Verification items for the finished model (mm, model axes). A direction names the side the tool comes from. Coordinates: 2 decimals unless noted, no trailing zeros. Loops run counter-clockwise (first coordinate to the right, second up) from the corner with the lowest first, then second, coordinate; pieces in that order, holes last.
Q1. Go/stop test with flat-tipped pins: P1, Ø19.5, axis at x = -7.5, y = 12, coming from the -Z side; P2, Ø6, axis at x = 42, z = 45, coming from the +Y side; P3, Ø12, axis at x = 10, y = 7.5, coming from the +Z side. Record where each tip stops, or that it passes through.
Q2. Mould release check, pull along Y, two halves, no side actions. Record for faces 1 (the face through (52.598, -32, 32)), 2 (the face through (-48.03, -17.81, 48.24)), 3 (the face through (42, 30.4, 29)): +Y half, -Y half, draft (parallel to the pull), parting line (faces both ways), or undercut.
Q3. Sectioned sample at D-D (x = -43.5). Enter the section's corners in (y, z), then the cut area to 3 significant figures.
Q4. Material ranges on probe 1 along Y at (x, z) = (28, 30.4); probe 2 along Y at (x, z) = (12.5, 29.4); probe 3 along Y at (x, z) = (39, 27.5), recorded low to high.
Q5. Sectioned sample at C-C (z = 55). Enter the section's corners in (x, y).
Q6. Sectioned sample at B-B (y = -0.65). Enter the section's corners in (x, z), then the cut area to 3 significant figures.
Q7. Sectioned sample at A-A (x = -3). Enter the section's corners in (y, z).
Q8. Access from +Z, -Z, +X, -X, +Y, -Y to the whole of each face (thin tool, end or side, straight path). Record for faces 4 (the face through (-1, -32, 65)), 5 (the face through (-1, -6.3, 29)), 6 (the face through (25, 15, 29)).
```python
from build123d import *

# Parameters (mm, degrees)
EXTRUDE_7_DEPTH     = 65
SKETCH_6_W          = 4
SKETCH_6_H          = 4
EXTRUDE_10_DEPTH    = 65
SKETCH_7_W          = 4
SKETCH_7_H          = 42.3
EXTRUDE_11_DEPTH    = 92
SKETCH_8_R          = 11.5
CUT_EXTRUDE_2_DEPTH = 2
SKETCH_10_R         = 2.5
CUT_EXTRUDE_3_DEPTH = 2
SKETCH_11_R         = 1.5
CUT_EXTRUDE_6_DEPTH = 4
EXTRUDE_13_DEPTH    = 2
SKETCH_14_R         = 0.7
EXTRUDE_14_DEPTH    = 5


with BuildPart() as part:
    # 草图1 → 凸台-拉伸7 (new body)
    with BuildSketch(Plane.XY):
        Polygon((-50, -29), (-50, -30.5), (-52.598076211, -29), (-52.598076211, -34), (-50, -32.5), (-50, -35.5), (50, -35.5), (50, -32.5), (52.598076211, -34), (52.598076211, -29), (50, -30.5), (50, -29), align=None)
    extrude(amount=EXTRUDE_7_DEPTH)

    # 草图6 → 凸台-拉伸10 (add)
    with BuildSketch(Plane(origin=(0, -29, 0), x_dir=(1, 0, 0), z_dir=(0, 1, 0))):
        with Locations((-48, -29)):
            Rectangle(SKETCH_6_W, SKETCH_6_H)
    extrude_10 = extrude(amount=EXTRUDE_10_DEPTH)

    # 镜向1: 凸台-拉伸10 across plane
    add(extrude_10.mirror(Plane(origin=(0, 0, 0), x_dir=(0, 0, 1), z_dir=(1, 0, 0))))

    # 草图7 → 凸台-拉伸11 (add)
    with BuildSketch(Plane(origin=(-46, 0, 0), x_dir=(0, 0, -1), z_dir=(1, 0, 0))):
        with Locations((-29, 14.85)):
            Rectangle(SKETCH_7_W, SKETCH_7_H)
    extrude(amount=EXTRUDE_11_DEPTH)

    # 草图8 → 切除-拉伸2 (cut)
    with BuildSketch(Plane.XY.offset(31)):
        with Locations((-28, 14.85)):
            Circle(SKETCH_8_R)
        with Locations((28, 14.85)):
            Circle(SKETCH_8_R)
    extrude(amount=-CUT_EXTRUDE_2_DEPTH, mode=Mode.SUBTRACT)

    # 草图10 → 切除-拉伸3 (cut)
    with BuildSketch(Plane.XY.offset(29)):
        with Locations((-28, 14.85)):
            Circle(SKETCH_10_R)
        with Locations((28, 14.85)):
            Circle(SKETCH_10_R)
    extrude(amount=-CUT_EXTRUDE_3_DEPTH, mode=Mode.SUBTRACT)

    # 草图11 → 切除-拉伸6 (cut)
    with BuildSketch(Plane.XY.offset(31)):
        with Locations((-43.5, 30.35)):
            Circle(SKETCH_11_R)
        with Locations((-12.5, 30.35)):
            Circle(SKETCH_11_R)
        with Locations((-43.5, -0.65)):
            Circle(SKETCH_11_R)
        with Locations((-12.5, -0.65)):
            Circle(SKETCH_11_R)
        with Locations((12.5, 30.35)):
            Circle(SKETCH_11_R)
        with Locations((43.5, 30.35)):
            Circle(SKETCH_11_R)
        with Locations((12.5, -0.65)):
            Circle(SKETCH_11_R)
        with Locations((43.5, -0.65)):
            Circle(SKETCH_11_R)
    extrude(amount=-CUT_EXTRUDE_6_DEPTH, mode=Mode.SUBTRACT)

    # 草图13 → 凸台-拉伸13 (add, symmetric)
    with BuildSketch(Plane(origin=(48, 0, 0), x_dir=(0, 0, -1), z_dir=(1, 0, 0))):
        Polygon((-65, -29), (-31, -6.3), (-31, -11.3), (-57.511013216, -29), align=None)
    extrude_13 = extrude(amount=EXTRUDE_13_DEPTH, both=True)

    # 镜向3: 凸台-拉伸13 across plane
    add(extrude_13.mirror(Plane(origin=(0, 0, 0), x_dir=(0, 0, 1), z_dir=(1, 0, 0))))

    # 草图14 → 凸台-拉伸14 (add)
    with BuildSketch(Plane(origin=(0, -29, 0), x_dir=(1, 0, 0), z_dir=(0, 1, 0))):
        with Locations(Location((-30.407474137, -14.090366943, 0), (0, 0, 180))):
            Circle(SKETCH_14_R)
        with Locations(Location((-31.677474137, -62.350366943, 0), (0, 0, 180))):
            Circle(SKETCH_14_R)
        with Locations(Location((20.392525863, -29.330366943, 0), (0, 0, 180))):
            Circle(SKETCH_14_R)
        with Locations(Location((20.392525863, -57.270366943, 0), (0, 0, 180))):
            Circle(SKETCH_14_R)
    extrude(amount=EXTRUDE_14_DEPTH)


solid = part.part
```
Geometry check:
1. P1: stops at z = 27
1. P2: stops at y = -29
1. P3: stops at z = 31
2. face 1: draft
2. face 2: +Y half
2. face 3: undercut
3. outline: (-35.5, 0) - (-29, 0) - (-29, 65) - (-35.5, 65) - close; (-6.3, 27) - (-2.15, 27) - (-2.15, 31) - (-6.3, 31) - close; (0.85, 27) - (28.85, 27) - (28.85, 31) - (0.85, 31) - close; (31.85, 27) - (36, 27) - (36, 31) - (31.85, 31) - close
3. area: 568 mm2
4. probe 1: y = -35.5 to -29, -6.3 to 3.35, 26.35 to 36
4. probe 2: y = -35.5 to -29, -6.3 to -2.15, 0.85 to 28.85, 31.85 to 36
4. probe 3: y = -35.5 to -29, -6.3 to 36
5. outline: (-52.6, -34) - (-50, -32.5) - (-50, -35.5) - (50, -35.5) - (50, -32.5) - (52.6, -34) - (52.6, -29) - (50, -30.5) - (50, -29) - (-50, -29) - (-50, -30.5) - (-52.6, -29) - close; (-50, -27.32) - (-46, -27.32) - (-46, -22.32) - (-50, -22.32) - close; (46, -27.32) - (50, -27.32) - (50, -22.32) - (46, -22.32) - close
6. outline: (-50, 27) - (-45, 27) - (-45, 31) - (-50, 31) - close; (-42, 27) - (-14, 27) - (-14, 31) - (-42, 31) - close; (-11, 27) - (11, 27) - (11, 31) - (-11, 31) - close; (14, 27) - (42, 27) - (42, 31) - (14, 31) - close; (45, 27) - (50, 27) - (50, 31) - (45, 31) - close
6. area: 352 mm2
7. outline: (-35.5, 0) - (-29, 0) - (-29, 65) - (-35.5, 65) - close; (-6.3, 27) - (36, 27) - (36, 31) - (-6.3, 31) - close
8. face 4: +Z, +X, -X, +Y, -Y
8. face 5: +Z, -Z
8. face 6: +Z
